Source: CAD feature listing. Evaluate the final solid. Frame: model axes, mm. A direction names the side the tool comes from. Coordinates: 2 decimals unless noted, no trailing zeros. Order: outer loops, then holes, each group sorted by start corner. A loop starts at its lowest first (then second) coordinate and runs counter-clockwise, first axis right, second up.
Autodesk Inventor part; units mm, degrees
ref_plane "YZ Plane" through (0, 0, 0) normal (1, 0, 0) x (0, 1, 0)
ref_plane "XZ Plane" through (0, 0, 0) normal (0, 1, 0) x (-1, 0, 0)
ref_plane "XY Plane" through (0, 0, 0) normal (0, 0, 1) x (1, 0, 0)
sketch "Sketch1" plane through (0, 0, 0) normal (0, 0, 1) x (1, 0, 0)
  point P0 (0, 0)
sketch "Sketch2" plane through (0, 0, 0) normal (0, 0, 1) x (1, 0, 0)
  circle A0 centre (0, 0) radius 3
  dimension "d0" = 6
extrude "Extrusion1" add sketch "Sketch2" along normal blind 10
sketch "Sketch3" plane through (0, 0, 10) normal (0, 0, 1) x (1, 0, 0)
  circle A0 centre (0, 0) radius 2
  dimension "d3" = 4
extrude "Extrusion2" add sketch "Sketch3" along normal blind 15
sketch "Sketch4" plane through (0, 0, 0) normal (0, 0, -1) x (-1, 0, 0)
  circle A0 centre (0, 0) radius 3
extrude "Extrusion3" add sketch "Sketch4" along normal blind 10
sketch "Sketch5" plane through (0, 0, -10) normal (0, 0, -1) x (-1, 0, 0)
  circle A0 centre (0, 0) radius 2
  circle A1 centre (0, 0) radius 3.5
  dimension "d8" = 7
extrude "Extrusion4" add sketch "Sketch5" against normal blind 1
sketch "Sketch6" plane through (0, 0, -9) normal (0, 0, 1) x (1, 0, 0)
  point P0 (0, 0)
sketch "Sketch7" plane through (0, 0, 10) normal (0, 0, 1) x (1, 0, 0)
  circle A0 centre (0, 0) radius 3
  circle A1 centre (0, 0) radius 2.925
  dimension "d11" = 5.85
extrude "Extrusion5" cut sketch "Sketch7" against normal up to surface (19 mm away)
fillet "Fillet1" radius 2 1 edges at (-2, 0, 10)
properties part number "Eje"
Q1. Pin query (flat end, axial travel): P1, Ø3, axis at x = -0.5, z = 11, coming from the +Y side (3 decimals); P2, Ø1.5, axis at y = 0, z = 5.5, coming from the -X side (3 decimals); P3, Ø3, axis at y = -1, z = 13, coming from the +X side. Return the tip coordinate at first contact, or that it passes through.
Solutions:
P1: stops at y = 2.925
P2: stops at x = -2.925
P3: stops at x = 2
Q2. Section query D-D on z = 17. Output: boundary loops of the cut face in (x, y), plus the area to 3 significant figures.
Solutions:
outline: circle Ø4 at (0, 0)
area: 12.6 mm2
Q3. Material intervals for line 1 along Y through (x, z) = (0, 21); line 2 along Z through (x, y) = (1, 3); line 3 along Y through (x, z) = (-0.25, 9.5), sorted ascending.
Solutions:
line 1: y = -2 to 2
line 2: z = -10 to -9
line 3: y = -2.91 to 2.91
Q4. Section query C-C on z = -1.5. Output: boundary loops of the cut face in (x, y) (3 decimals), plus the area to 3 significant figures.
Solutions:
outline: circle Ø5.85 at (0, 0)
area: 26.9 mm2
Q5. Section query A-A on x = 0. Output: boundary loops of the cut face in (y, z) (3 decimals), plus the area to 3 significant figures.
Solutions:
outline: (-3.5, -10) - (3.5, -10) - (3.5, -9) - (2.925, -9) - (2.925, 10) arc R2 cw to (2, 11.687) - (2, 25) - (-2, 25) - (-2, 11.687) arc R2 cw to (-2.925, 10) - (-2.925, -9) - (-3.5, -9) - close
area: 179 mm2
Q6. Set-up query: faces 1 (the flat face through (0, 0, 25)), 2 (the cylindrical face through (-0.634, -2.855, 0.633)). Return all of +Z, -Z, +X, -X, +Y, -Y with unobstructed straight access to the full face (end or side cutting, diameter ignored); none if empty.
Solutions:
face 1: +Z, +X, -X, +Y, -Y
face 2: +Z
